from build123d import *

# Parameters (mm, degrees)
F1_DEPTH = 0.8
F2_W     = 76.2
F2_H     = 213.36
F2_W_2   = 36.9
F2_H_2   = 211.76
F3_DEPTH = 44
F4_DEPTH = 0.8


with BuildPart() as f1:
    # F0 (on Top) → F1 (new body)
    with BuildSketch(Plane.XY):
        with BuildLine():
            ThreePointArc((0, 12.5), (8.838835, 8.838835), (12.5, 0))
            Line((12.5, 0), (63.7, 0))
            ThreePointArc((63.7, 0), (67.361165, 8.838835), (76.2, 12.5))
            Line((76.2, 12.5), (76.2, 200.86))
            ThreePointArc((76.2, 200.86), (67.361165, 204.521165), (63.7, 213.36))
            Line((63.7, 213.36), (12.5, 213.36))
            ThreePointArc((12.5, 213.36), (8.838835, 204.521165), (0, 200.86))
            Line((0, 200.86), (0, 12.5))
        make_face()
        with BuildLine():
            Line((0, 12.5), (0, 0))
            Line((0, 0), (12.5, 0))
            ThreePointArc((12.5, 0), (8.838835, 8.838835), (0, 12.5))
        make_face()
        with BuildLine():
            ThreePointArc((63.7, 213.36), (67.361165, 204.521165), (76.2, 200.86))
            Line((76.2, 200.86), (76.2, 213.36))
            Line((76.2, 213.36), (63.7, 213.36))
        make_face()
        with BuildLine():
            Line((0, 213.36), (0, 200.86))
            ThreePointArc((0, 200.86), (8.838835, 204.521165), (12.5, 213.36))
            Line((12.5, 213.36), (0, 213.36))
        make_face()
    extrude(amount=F1_DEPTH)

    # F2 (on face) → F3 (join)
    with BuildSketch(Plane.XY.offset(0.8)):
        with Locations((38.1, 106.68)):
            Rectangle(F2_W, F2_H)
        with Locations((19.25, 106.68)):
            Rectangle(F2_W_2, F2_H_2, mode=Mode.SUBTRACT)
        with Locations((56.95, 106.68)):
            Rectangle(F2_W_2, F2_H_2, mode=Mode.SUBTRACT)
    extrude(amount=F3_DEPTH)

    # F0 (on Top) → F4 (join, through all)
    with BuildSketch(Plane.XY):
        with BuildLine():
            Line((76.2, 0), (63.7, 0))
            ThreePointArc((63.7, 0), (76.2, -12.5), (88.7, 0))
            ThreePointArc((88.7, 0), (85.038835, 8.838835), (76.2, 12.5))
            Line((76.2, 12.5), (76.2, 0))
        make_face()
        with BuildLine():
            Line((12.5, 0), (0, 0))
            Line((0, 0), (0, 12.5))
            ThreePointArc((0, 12.5), (-8.838835, -8.838835), (12.5, 0))
        make_face()
        with BuildLine():
            ThreePointArc((12.5, 213.36), (-8.838835, 222.198835), (0, 200.86))
            Line((0, 200.86), (0, 213.36))
            Line((0, 213.36), (12.5, 213.36))
        make_face()
        with BuildLine():
            Line((76.2, 213.36), (76.2, 200.86))
            ThreePointArc((76.2, 200.86), (85.038835, 204.521165), (88.7, 213.36))
            ThreePointArc((88.7, 213.36), (76.2, 225.86), (63.7, 213.36))
            Line((63.7, 213.36), (76.2, 213.36))
        make_face()
        with BuildLine():
            ThreePointArc((76.2, 12.5), (67.361165, 8.838835), (63.7, 0))
            Line((63.7, 0), (76.2, 0))
            Line((76.2, 0), (76.2, 12.5))
        make_face()
        with BuildLine():
            Line((0, 12.5), (0, 0))
            Line((0, 0), (12.5, 0))
            ThreePointArc((12.5, 0), (8.838835, 8.838835), (0, 12.5))
        make_face()
        with BuildLine():
            Line((0, 213.36), (0, 200.86))
            ThreePointArc((0, 200.86), (8.838835, 204.521165), (12.5, 213.36))
            Line((12.5, 213.36), (0, 213.36))
        make_face()
        with BuildLine():
            ThreePointArc((63.7, 213.36), (67.361165, 204.521165), (76.2, 200.86))
            Line((76.2, 200.86), (76.2, 213.36))
            Line((76.2, 213.36), (63.7, 213.36))
        make_face()
    extrude(amount=F4_DEPTH)


solid = f1.part
The model under review builds one solid part; all positions refer to its coordinate system, in mm. A direction names the side the tool comes from. Round coordinates to 2 decimals unless told otherwise and drop trailing zeros. Order: outer loops, then holes, each group sorted by start corner. A loop starts at its lowest first (then second) coordinate and runs counter-clockwise, first axis right, second up. Notation, with made-up numbers: (21.5, 40.5) -> (56.5, 40.5) arc R12 ccw to (56.5, 62.5) -> close; hole circle Ø8 at (22.5, 11.5). An arc over 180 degrees is marked (long way). Use CSV: the item, a comma, the result in double quotes. Start each with the question number.
(1) Consider section D-D on y = 204.5. Write out the cut boundary in (x, z), and give its area (3 significant figures).
(2) Mouldability with a two-part tool opening along X and no side actions: class faces 1 (the face through (0, 214, 0.8)), 2 (the face through (38.5, 105, 22)), 3 (the face through (75.4, 105, 22)), 4 (the face through (0, 105, 22)) as pulls with the +X half, pulls with the -X half, needs draft (parallel to the pull), parting line crosses it, or undercut.
(3) Wall thickness on probe 1 along X at (y, z) = (203, 13); probe 2 along Y at (x, z) = (65.5, 23); probe 3 along Z at (x, y) = (62, 205): over which ranges is each line inside the solid? List them lowest first. Write a range as from..to.
(4) Consider section C-C on x = 27.5. Write out the cut boundary in (y, z).
(5) Tool access review of faces 5 (the face through (-9.13, -8.54, 0.39)), 6 (the face through (19, 108, 0.8)): name each direction out of +Z, -Z, +X, -X, +Y, -Y from which nothing blocks a thin tool from reaching the whole face with its end or side.
(6) Consider section B-B on z = 4. Write out the cut boundary in (x, y).
(7) Insertion check: pin 1 (10 mm diameter, centred on y = 14.5, z = 15.5, fed in from -X); pin 2 (18.5 mm diameter, centred on x = 66, z = 23, fed in from +Y); pin 3 (18.5 mm diameter, centred on x = 21, z = 28.5, fed in from -Y). Each pin has a flat end and moves straight along its axis. Give the tip position at first contact, or say it passes through.
(8) Consider section A-A on y = 142. Write out the cut boundary in (x, z).
Responses:
1,outline,"(-8.82, 0) -> (85.02, 0) -> (85.02, 0.8) -> (76.2, 0.8) -> (76.2, 44.8) -> (75.4, 44.8) -> (75.4, 0.8) -> (38.5, 0.8) -> (38.5, 44.8) -> (37.7, 44.8) -> (37.7, 0.8) -> (0.8, 0.8) -> (0.8, 44.8) -> (0, 44.8) -> (0, 0.8) -> (-8.82, 0.8) -> close"
1,area,"181 mm²"
2,face 1,"needs draft"
2,face 2,"undercut"
2,face 3,"undercut"
2,face 4,"pulls with the -X half"
3,probe 1,"0..0.8, 37.7..38.5, 75.4..76.2"
3,probe 2,"0..0.8, 212.56..213.36"
3,probe 3,"0..0.8"
4,outline,"(0, 0) -> (213.36, 0) -> (213.36, 44.8) -> (212.56, 44.8) -> (212.56, 0.8) -> (0.8, 0.8) -> (0.8, 44.8) -> (0, 44.8) -> close"
5,face 5,"+Z, -Z"
5,face 6,"+Z"
6,outline,"(0, 0) -> (76.2, 0) -> (76.2, 213.36) -> (0, 213.36) -> close; hole (0.8, 0.8) -> (37.7, 0.8) -> (37.7, 212.56) -> (0.8, 212.56) -> close; hole (38.5, 0.8) -> (75.4, 0.8) -> (75.4, 212.56) -> (38.5, 212.56) -> close"
7,pin 1,"x = 0"
7,pin 2,"y = 213.36"
7,pin 3,"y = 0"
8,outline,"(0, 0) -> (76.2, 0) -> (76.2, 44.8) -> (75.4, 44.8) -> (75.4, 0.8) -> (38.5, 0.8) -> (38.5, 44.8) -> (37.7, 44.8) -> (37.7, 0.8) -> (0.8, 0.8) -> (0.8, 44.8) -> (0, 44.8) -> close"
